Can you work these out from the model? Positions are in its coordinate system, mm. Face numbers are marked on the shaded views. A direction names the side the tool comes from. Round coordinates to 2 decimals unless told otherwise and drop trailing zeros. Loops run counter-clockwise (first coordinate to the right, second up) from the corner with the lowest first, then second, coordinate; pieces in that order, holes last.
from build123d import *

# Parameters (mm, degrees)
F2_R     = 1.6
F3_DEPTH = 15
F5_DEPTH = 15


with BuildPart() as f1:
    # F0 (on Front) → F1 (revolve)
    with BuildSketch(Plane.XZ):
        Polygon((0, 15), (0, 0), (5, 0), (4, 15), align=None)
    revolve(axis=Axis((0, 0, 7.5), (0, 0, -1)))

    # F2 (on face) → F3 (cut, through all)
    with BuildSketch(Plane.XY.offset(15)):
        Circle(F2_R)
    extrude(amount=-F3_DEPTH, mode=Mode.SUBTRACT)

    # F4 (on face) → F5 (join, through all)
    with BuildSketch(Plane.XY.offset(15)):
        with BuildLine():
            ThreePointArc((0.3180668057, 1.5680668057), (0, 1.6), (-0.3180668057, 1.5680668057))
            Line((-0.3180668057, 1.5680668057), (0, 1.25))
            Line((0, 1.25), (0.3180668057, 1.5680668057))
        make_face()
        with BuildLine():
            ThreePointArc((1.1989522857, -1.0594873367), (1.3856406461, -0.8), (1.5170190914, -0.508579469))
            Line((1.5170190914, -0.508579469), (1.0825317547, -0.625))
            Line((1.0825317547, -0.625), (1.1989522857, -1.0594873367))
        make_face()
        with BuildLine():
            Line((-1.0825317547, -0.625), (-1.5170190914, -0.508579469))
            ThreePointArc((-1.5170190914, -0.508579469), (-1.3856406461, -0.8), (-1.1989522857, -1.0594873367))
            Line((-1.1989522857, -1.0594873367), (-1.0825317547, -0.625))
        make_face()
    extrude(amount=-F5_DEPTH)


solid = f1.part
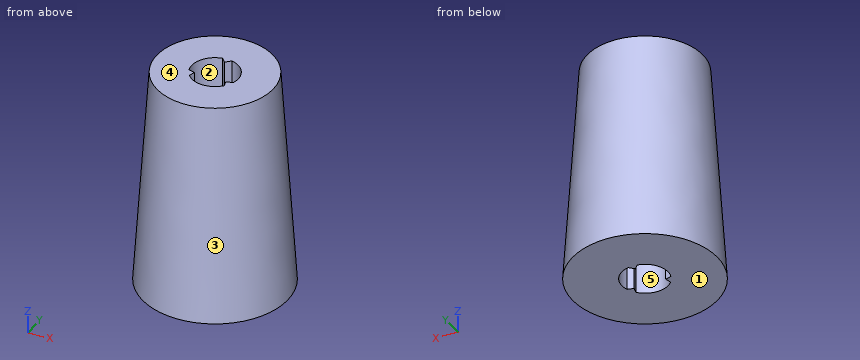
(1) For the marked faces 1 and 2, which set-ups out of +Z, -Z, +X, -X, +Y, -Y let a thin tool reach every point of the face, with its end or its side?
Worked answers:
face 1: -Z, +X, -X, +Y, -Y
face 2: +Z, -Z
(2) If we mould it in two halves opening along X, with no side actions, what happens to the marked faces 3, 4 and 5? For each: released by +X, released by -X, zero draft, split by the parting line, or undercut.
Worked answers:
face 3: split by the parting line
face 4: zero draft
face 5: undercut
(3) If I drill on line 1 (Y direction, x = 1, z = 1.5); line 2 (X direction, y = -1, z = 11.25); line 3 (X direction, y = -1.25, z = 9.75), over which ranges is the centre line in solid material (lowest first)?
Worked answers:
line 1: y = -4.8 to -1.25, 1.25 to 4.8
line 2: x = -4.13 to -1.18, 1.18 to 4.13
line 3: x = -4.17 to -1, 1 to 4.17
(4) If we section it at A-A, the plane z = 6.75: List the corners of the cut face in (x, y) for me (3 decimals), then the cut area to 3 significant figures.
Worked answers:
outline: circle Ø9.1 at (0, 0); hole (-1.517, -0.509) - (-1.083, -0.625) - (-1.199, -1.059) arc R1.6 ccw to (1.199, -1.059) - (1.083, -0.625) - (1.517, -0.509) arc R1.6 ccw to (0.318, 1.568) - (0, 1.25) - (-0.318, 1.568) arc R1.6 ccw to start
area: 57.3 mm2
(5) If we section it at C-C, the plane z = 9.75: List the corners of the cut face in (x, y) for me (3 decimals).
Worked answers:
outline: circle Ø8.7 at (0, 0); hole (-1.517, -0.509) - (-1.083, -0.625) - (-1.199, -1.059) arc R1.6 ccw to (1.199, -1.059) - (1.083, -0.625) - (1.517, -0.509) arc R1.6 ccw to (0.318, 1.568) - (0, 1.25) - (-0.318, 1.568) arc R1.6 ccw to start
(6) Will these pins go through, and if not, where does the flat tip stop? P1, Ø5, axis at y = 4, z = 5, coming from the -X side; P2, Ø1, axis at y = 4, z = 3, coming from the -X side; P3, Ø2, axis at x = 0.5, z = 7, coming from the +Y side.
Worked answers:
P1: stops at x = -4.44
P2: stops at x = -3.29
P3: stops at y = 4.59
(7) If we section it at B-B, the plane y = 0: List the corners of the cut face in (x, z) for me, then the cut area to 3 significant figures.
Worked answers:
outline: (-5, 0) - (-1.6, 0) - (-1.6, 15) - (-4, 15) - close; (1.6, 0) - (5, 0) - (4, 15) - (1.6, 15) - close
area: 87.0 mm2
